Model file for the job. Use its own axes, mm. Face numbers are marked on the shaded views. Round coordinates to 2 decimals unless told otherwise and drop trailing zeros. Order: outer loops, then holes, each group sorted by start corner. A loop starts at its lowest first (then second) coordinate and runs counter-clockwise, first axis right, second up. Notation, with made-up numbers: (20, 38.5) - (48, 38.5) arc R28 ccw to (48, 56.5) - close; hole circle Ø10 at (4, 56). An arc over 180 degrees is marked (long way). Use one line per item in the form item = value.
Autodesk Inventor part; units mm, degrees
ref_plane "YZ Plane" through (0, 0, 0) normal (1, 0, 0) x (0, 1, 0)
ref_plane "XZ Plane" through (0, 0, 0) normal (0, 1, 0) x (-1, 0, 0)
ref_plane "XY Plane" through (0, 0, 0) normal (0, 0, 1) x (1, 0, 0)
sketch "Sketch1" plane through (0, 0, 0) normal (0, 0, 1) x (1, 0, 0)
  circle A0 centre (0, 0) radius 20
  circle A1 centre (0, 0) radius 23
  dimension "d0" = 40
  dimension "d1" = 46
extrude "Extrusion1" add sketch "Sketch1" along normal mid plane 178
sketch "Sketch2" plane through (0, 0, 0) normal (1, 0, 0) x (0, 1, 0)
  line L0 (0, 70) -> (0, -70)
  line L1 (-70, 0) -> (70, 0)
  point P0 (0, 0)
  point P1 (0, 35)
  point P2 (0, -35)
  dimension "d19" = 35
  dimension "d20" = 70
hole "Hole1" at (0, 0, 35) at (0, 0, -35) direction (-1, 0, 0) diameter 4.5 end through all
sketch "Sketch3" plane through (0, 0, 0) normal (1, 0, 0) x (0, 1, 0)
  line L0 (23, -89) -> (7, -89)
  line L1 (7, -89) -> (7, 89)
  line L2 (7, 89) -> (23, 89)
  line L3 (23, 89) -> (23, -89)
  line L4 (23, 89) -> (-23, 89)
  line L5 (-23, -89) -> (23, -89)
  line L6 (0, 159.6) -> (0, -159.6)
  point P0 (0, 0)
  dimension "d13" = 0
  dimension "d14" = 0
  dimension "d15" = 7
extrude "Extrusion2" cut sketch "Sketch3" along normal through all both and the other way through all contours L0 L1 L2 L3
properties part number "Top_Tilt Pipe_3 Lanes" material "PVC-Piping"
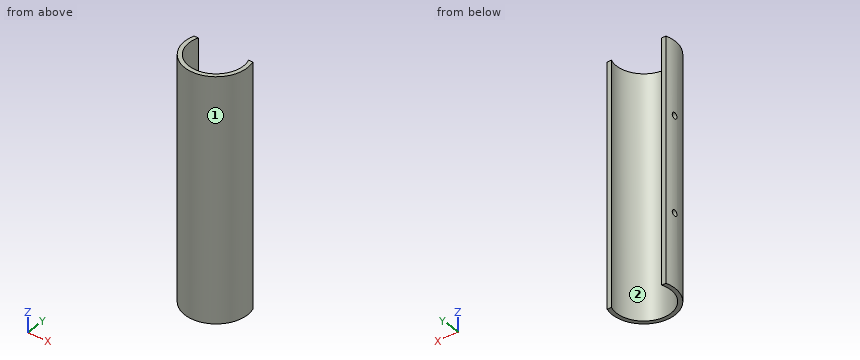
(1) Probe probe 1 along Z at (x, y) = (-21.1, 0); probe 2 along X at (y, z) = (-7, -24) (3 decimals); probe 3 along X at (y, z) = (0, -2). List the from-to ranges inside material, lowest first. Write a range as [from, to].
Report:
probe_1 = [-89, -37.25], [-32.75, 32.75], [37.25, 89]
probe_2 = [-21.909, -18.735], [18.735, 21.909]
probe_3 = [-23, -20], [20, 23]
(2) Slice it at D-D on x = 0. Give the cut face in (y, z), then the cut area to 3 significant figures.
Report:
outline = (-23, -89) - (-20, -89) - (-20, 89) - (-23, 89) - close
area = 534 mm2
(3) Pull direction X, two halves, no side cores. Call the marked faces 1 and 2: released by +X, released by -X, zero draft, split by the parting line, or undercut.
Report:
face_1 = split by the parting line
face_2 = undercut
(4) Slice it at C-C on y = -17. Give the cut face in (x, z).
Report:
outline = (-15.49, -89) - (-10.54, -89) - (-10.54, 89) - (-15.49, 89) - close; (10.54, -89) - (15.49, -89) - (15.49, 89) - (10.54, 89) - close
(5) Pin check, flat tips, straight feed: pin 1 (4 mm diameter, centred on x = 15, z = -35.5, fed in from +Y); pin 2 (1 mm diameter, centred on x = 2.5, z = -26.5, fed in from +Y); pin 3 (1 mm diameter, centred on y = -9, z = 39, fed in from -X); pin 4 (12 mm diameter, centred on x = 8.5, y = -1, fed in from -Z). Stop position of each tip, or through.
Report:
pin_1 = -10.54
pin_2 = -19.77
pin_3 = -21.37
pin_4 = through
(6) Slice it at B-B on z = -35. Give the cut face in (x, y) (3 decimals).
Report:
outline = (-22.89, -2.25) arc R23 ccw (long way) to (21.909, 7) - (18.735, 7) arc R20 cw (long way) to (-19.873, -2.25) - close; (-22.89, 2.25) - (-19.873, 2.25) arc R20 cw to (-18.735, 7) - (-21.909, 7) arc R23 ccw to start
(7) Slice it at A-A on y = 0. Give the cut face in (x, z), then the cut area to 3 significant figures.
Report:
outline = (-23, -89) - (-20, -89) - (-20, -37.25) - (-23, -37.25) - close; (-23, -32.75) - (-20, -32.75) - (-20, 32.75) - (-23, 32.75) - close; (-23, 37.25) - (-20, 37.25) - (-20, 89) - (-23, 89) - close; (20, -89) - (23, -89) - (23, 89) - (20, 89) - close
area = 1,040 mm2
